The model under review builds one solid part; all positions refer to its coordinate system, in mm. A direction names the side the tool comes from. Round coordinates to 2 decimals unless told otherwise and drop trailing zeros. Loops run counter-clockwise (first coordinate to the right, second up) from the corner with the lowest first, then second, coordinate; pieces in that order, holes last. Notation, with made-up numbers: M 72.25,-12 L 125.25,-12 A30 ccw 125.25,17 Z; hole C 8,-9.5 d8. An arc over 180 degrees is marked long. Answer as a JSON object with one key per item and string values. Group by question number.
Item 1: The part is to be moulded in two halves that separate along X. For faces 4 (the face through (-19.8, 31.4, 5.5)), 5 (the face through (-56.828, 0.634, 1.905)), 6 (the face through (-7, -8, 11.176)), 7 (the face through (-1.542, -0.044, 24.569)), say which applies: +X half, -X half, draft (parallel to the pull), parting line (faces both ways), or undercut.
Item 2: Consider section B-B (y = 27). Give the boundary of the cut face in (x, z), and give its area (3 significant figures).
Item 3: Consider section D-D (z = 34.5). Give the boundary of the cut face in (x, y) (1 decimal).
Item 4: Insertion check: P1, Ø5, axis at x = -14, y = -14.5, coming from the +Z side; P2, Ø5, axis at y = -9.5, z = 15.5, coming from the +X side; P3, Ø6, axis at y = -17, z = 19, coming from the +X side; P4, Ø23, axis at x = -42.43, y = 0, coming from the -Z side. Each pin has a flat end and moves straight along its axis. Give the tip position at first contact, or say it passes through.
Item 5: To check wall thickness, follow line 1 (Y direction, x = 10, z = 5.5); line 2 (Z direction, x = 14, y = -25); line 3 (Y direction, x = -36, z = 6). State the ranges of each line that lie inside material, in increasing order.
Item 6: Consider section A-A (z = 10). State how many separate pieces and enclosed holes the cut face has, and give its area (3 significant figures).
Item 7: Consider section C-C (x = 10). Give the boundary of the cut face in (y, z) (3 decimals).
Item 8: Tool access review of faces 1 (the face through (-8, 3.175, 18)), 2 (the face through (-5, -3.175, 21)), 3 (the face through (7.55, -22.28, 5.51)): name each direction out of +Z, -Z, +X, -X, +Y, -Y from which nothing blocks a thin tool from reaching the whole face with its end or side.
```python
from build123d import *

# Parameters (mm, degrees)
F0_R     = 14.2875
F1_DEPTH = 41.148
F0_R_2   = 6.35
F2_DEPTH = 11.176
F3_DEPTH = 37.592
F5_DEPTH = 127
F6_DEPTH = 76.2
F7_R     = 3.048
F8_SIZE2 = 2.032
F8_SIZE  = 2.032
F9_SIZE2 = 2.032
F9_SIZE  = 2.032


# Not quite as in the source:
# - ends of sketch curves that miss each other by under 0.0002 mm in the source are joined


with BuildPart() as f1:
    # F0 (on Top) → F1 (new body)
    with BuildSketch(Plane.XY):
        with BuildLine():
            ThreePointArc((-17.226482478, 3.175), (-26.6125443992, 19.8759818106), (-44.9953409853, 25.2698432749))
            ThreePointArc((-44.9953409853, 25.2698432749), (-67.8272637159, 0), (-44.9953409853, -25.2698432749))
            ThreePointArc((-44.9953409853, -25.2698432749), (-26.6125443992, -19.8759818106), (-17.226482478, -3.175))
            Line((-17.226482478, -3.175), (-23.8334226287, -3.175))
            Line((-23.8334226287, -3.175), (-23.8334226287, 3.175))
            Line((-23.8334226287, 3.175), (-17.226482478, 3.175))
        make_face()
        with Locations((-42.4272637159, 0)):
            Circle(F0_R, mode=Mode.SUBTRACT)
        with BuildLine():
            ThreePointArc((-17.0272637159, 0), (-17.0771173313, 1.5906219786), (-17.226482478, 3.175))
            Line((-17.226482478, 3.175), (-23.8334226287, 3.175))
            Line((-23.8334226287, 3.175), (-23.8334226287, -3.175))
            Line((-23.8334226287, -3.175), (-17.226482478, -3.175))
            ThreePointArc((-17.226482478, -3.175), (-17.0771173313, -1.5906219786), (-17.0272637159, 0))
        make_face()
    extrude(amount=F1_DEPTH)

    # F0 (on Top) → F2 (join)
    with BuildSketch(Plane.XY):
        with BuildLine():
            Line((4.6864668266, 37.3577696364), (-44.9953409853, 25.2698432749))
            ThreePointArc((-44.9953409853, 25.2698432749), (-26.6125443992, 19.8759818106), (-17.226482478, 3.175))
            Line((-17.226482478, 3.175), (14.5881694606, 3.175))
            Line((14.5881694606, 3.175), (14.5881694606, -3.175))
            Line((14.5881694606, -3.175), (-17.226482478, -3.175))
            ThreePointArc((-17.226482478, -3.175), (-26.6125443992, -19.8759818106), (-44.9953409853, -25.2698432749))
            Line((-44.9953409853, -25.2698432749), (6.0998825197, -37.8248519321))
            ThreePointArc((6.0998825197, -37.8248519321), (2.2878291463, -21.247003676), (17.8827435435, -28.0407838216))
            Line((17.8827435435, -28.0407838216), (17.8977366181, 28.575))
            ThreePointArc((17.8977366181, 28.575), (3.0995063243, 20.6428709799), (4.6864668266, 37.3577696364))
        make_face()
        with BuildLine():
            ThreePointArc((17.8827435435, -28.0407838216), (2.2878291463, -21.247003676), (6.0998825197, -37.8248519321))
            ThreePointArc((6.0998825197, -37.8248519321), (14.2496697061, -36.0708174039), (17.8977362841, -28.575))
            ThreePointArc((17.8977362841, -28.575), (17.8939873612, -28.307786739), (17.8827435435, -28.0407838216))
        make_face()
        with Locations((8.3727362841, -28.575)):
            Circle(F0_R_2, mode=Mode.SUBTRACT)
        with BuildLine():
            ThreePointArc((4.6864668266, 37.3577696364), (3.0995063243, 20.6428709799), (17.8977362841, 28.575))
            ThreePointArc((17.8977362841, 28.575), (13.6459662439, 36.5071290201), (4.6864668266, 37.3577696364))
        make_face()
        with Locations((8.3727362841, 28.575)):
            Circle(F0_R_2, mode=Mode.SUBTRACT)
        with BuildLine():
            Line((14.5881694606, 3.175), (-17.226482478, 3.175))
            ThreePointArc((-17.226482478, 3.175), (-17.0771173313, 1.5906219786), (-17.0272637159, 0))
            ThreePointArc((-17.0272637159, 0), (-17.0771173313, -1.5906219786), (-17.226482478, -3.175))
            Line((-17.226482478, -3.175), (14.5881694606, -3.175))
            Line((14.5881694606, -3.175), (14.5881694606, 3.175))
        make_face()
        with Locations((8.3727362841, 28.575)):
            Circle(F0_R_2)
        with Locations((8.3727362841, -28.575)):
            Circle(F0_R_2)
        with BuildLine():
            ThreePointArc((-17.0272637159, 0), (-17.0771173313, 1.5906219786), (-17.226482478, 3.175))
            Line((-17.226482478, 3.175), (-23.8334226287, 3.175))
            Line((-23.8334226287, 3.175), (-23.8334226287, -3.175))
            Line((-23.8334226287, -3.175), (-17.226482478, -3.175))
            ThreePointArc((-17.226482478, -3.175), (-17.0771173313, -1.5906219786), (-17.0272637159, 0))
        make_face()
    extrude(amount=F2_DEPTH)

    # F0 (on Top) → F3 (join)
    with BuildSketch(Plane.XY):
        with BuildLine():
            Line((14.5881694606, 3.175), (-17.226482478, 3.175))
            ThreePointArc((-17.226482478, 3.175), (-17.0771173313, 1.5906219786), (-17.0272637159, 0))
            ThreePointArc((-17.0272637159, 0), (-17.0771173313, -1.5906219786), (-17.226482478, -3.175))
            Line((-17.226482478, -3.175), (14.5881694606, -3.175))
            Line((14.5881694606, -3.175), (14.5881694606, 3.175))
        make_face()
    extrude(amount=F3_DEPTH)

    # F4 (on face) → F5 (cut)
    with BuildSketch(Plane.XZ.offset(3.175)):
        Polygon((14.5881694606, 37.592), (-17.226482478, 37.592), (14.5881694606, 11.176), align=None)
    extrude(amount=-F5_DEPTH, mode=Mode.SUBTRACT)

    # F0 (on Top) → F6 (cut)
    with BuildSketch(Plane.XY):
        with Locations((8.3727362841, 28.575)):
            Circle(F0_R_2)
        with Locations((8.3727362841, -28.575)):
            Circle(F0_R_2)
    extrude(amount=F6_DEPTH, mode=Mode.SUBTRACT)

    # F7
    f7_edges = [f1.edges().sort_by_distance(p)[0] for p in [
        (-39.859186, -25.269843, 41.148),
    ]]
    fillet(f7_edges, radius=F7_R)

    # F8
    f8_edges = [f1.edges().sort_by_distance(p)[0] for p in [
        (-56.714764, 0, 41.148),
        (-40.167356, -22.237462, 41.148),
    ]]
    chamfer(f8_edges, length=F8_SIZE, length2=F8_SIZE2)

    # F9
    f9_edges = [f1.edges().sort_by_distance(p)[0] for p in [
        (-56.714764, 0, 0),
    ]]
    chamfer(f9_edges, length=F9_SIZE, length2=F9_SIZE2)


solid = f1.part
```
Geometry results:
{
 "1": {"face 4": "-X half", "face 5": "undercut", "face 6": "draft", "face 7": "+X half"},
 "2": {"outline": "M -37.88,0 L 2.22,0 L 2.22,11.18 L -37.88,11.18 Z; M 14.52,0 L 17.9,0 L 17.9,11.18 L 14.52,11.18 Z", "area": "486 mm^2"},
 "3": {"outline": "M -17.2,-3.2 L -13.5,-3.2 L -13.5,3.2 L -17.2,3.2 A25.4 ccw long Z; hole C -42.4,0 d28.6"},
 "4": {"P1": "stops at z = 11.18", "P2": "stops at x = -18.01", "P3": "stops at x = -21.23", "P4": "passes through"},
 "5": {"line 1": "y = -37.96 to -34.71, -22.44 to 22.44, 34.71 to 37.96", "line 2": "z = 0 to 11.18", "line 3": "y = -27.48 to -12.76, 12.76 to 27.46"},
 "6": {"separate pieces": "1", "enclosed holes": "3", "area": "4,070 mm^2"},
 "7": {"outline": "M -37.96,0 L -34.713,0 L -34.713,11.176 L -37.96,11.176 Z; M -22.437,0 L 22.437,0 L 22.437,11.176 L 3.175,11.176 L 3.175,14.986 L -3.175,14.986 L -3.175,11.176 L -22.437,11.176 Z; M 34.713,0 L 37.96,0 L 37.96,11.176 L 34.713,11.176 Z"},
 "8": {"face 1": "+Z, +X, +Y", "face 2": "+Z, +X, -Y", "face 3": "+Z, -Z"}
}
